Part model, mm, in its own coordinate system. A direction names the side the tool comes from. Coordinates: 2 decimals unless noted, no trailing zeros. Loops run counter-clockwise (first coordinate to the right, second up) from the corner with the lowest first, then second, coordinate; pieces in that order, holes last. Notation, with made-up numbers: (41.25, 20.25) - (55.25, 20.25) arc R35 ccw to (55.25, 58.25) - close; hole circle Ø4 at (-23.5, 49.5). An arc over 180 degrees is marked (long way). Use a Markdown table: item, result. Add a question column.
1. Band-saw the part on D-D, the plane x = 13. Give the cut face in (y, z).
2. Band-saw the part on C-C, the plane z = 9. Give the cut face in (x, y), plus the area to 3 significant figures.
3. Drop flat-ended pins along their axis: pin 1 (10 mm diameter, centred on y = -2, z = 5.5, fed in from -X); pin 2 (10 mm diameter, centred on x = -1, z = -10, fed in from -Y); pin 3 (1 mm diameter, centred on x = -7.5, z = -18.5, fed in from +Y); pin 4 (8 mm diameter, centred on y = -5.5, z = 2.5, fed in from -X). Give the stop position or say it passes through.
4. Band-saw the part on B-B, the plane y = -2. Give the cut face in (x, z), plus the area to 3 significant figures.
5. Band-saw the part on A-A, the plane x = -13. Give the cut face in (y, z), plus the area to 3 significant figures.
6. 3-axis set-ups, long thin cutter, end or side, ignore diameter. For faces 1 (the cylindrical face through (-15.95, -24.3, 18.51)), 2 (the flat face through (10, 1, 0)), 3 (the flat face through (-10, -7, 19)): which of +Z, -Z, +X, -X, +Y, -Y reach the whole face in a straight line?
7. Wall check: probe 1 along Y at (x, z) = (13, -18); probe 2 along Z at (x, y) = (1, -6); probe 3 along Y at (x, z) = (18, -17). Give the ranges that are in metal, low to high. Write a range as [from, to].
8. Pull direction Y, two halves, no side cores. Call faces 4 (the flat face through (0, -37, -18)), 5 (the flat face through (-5, 1.4, 4.4)), 6 (the cylindrical face through (12.479, -23.034, -18.486)), 7 (the flat face through (10, 3, 0)): pulls with the +Y half, pulls with the -Y half, needs draft (parallel to the pull), parting line crosses it, or undercut.
from build123d import *

# Parameters (mm, degrees)
HEAD_W_DEPTH        = 19.5
HEAD_T_W            = 35
HEAD_T_H            = 38
CUT_EXTRUDE_1_DEPTH = 66.186271561
SKETCH_3_R          = 4
CUT_EXTRUDE_2_DEPTH = 60.287435431


with BuildPart() as part:
    # ｽｹｯﾁ1 → Head-W (new, symmetric)
    with BuildSketch(Plane.XY):
        Polygon((-25, -37), (25, -37), (25, 3), (-5, 3), (-5, -7), (-15, -7), (-15, 3), (-25, 3), align=None)
    extrude(amount=HEAD_W_DEPTH, both=True)

    # Head-t → ｶｯﾄ - 押し出し1 (cut, through all)
    with BuildSketch(Plane(origin=(25, 0, 0), x_dir=(0, 0, -1), z_dir=(1, 0, 0))):
        with Locations((0, -18)):
            Rectangle(HEAD_T_W, HEAD_T_H)
    extrude(amount=-CUT_EXTRUDE_1_DEPTH, mode=Mode.SUBTRACT)

    # ｽｹｯﾁ3 → ｶｯﾄ - 押し出し2 (cut, through all)
    with BuildSketch(Plane.XY.offset(19.5)):
        with Locations((-13, -27)):
            Circle(SKETCH_3_R)
        with Locations((13, -27)):
            Circle(SKETCH_3_R)
    extrude(amount=-CUT_EXTRUDE_2_DEPTH, mode=Mode.SUBTRACT)


solid = part.part
Geometry check:
| question | item | result |
|---|---|---|
| 1 | outline | (-37, -19.5) - (-31, -19.5) - (-31, -17.5) - (-37, -17.5) - close; (-37, 17.5) - (-31, 17.5) - (-31, 19.5) - (-37, 19.5) - close; (-23, -19.5) - (3, -19.5) - (3, 19.5) - (-23, 19.5) - (-23, 17.5) - (1, 17.5) - (1, -17.5) - (-23, -17.5) - close |
| 2 | outline | (-25, 1) - (-15, 1) - (-15, 3) - (-25, 3) - close; (-5, 1) - (25, 1) - (25, 3) - (-5, 3) - close |
| 2 | area | 80.0 mm^2 |
| 3 | pin 1 | stops at x = -25 |
| 3 | pin 2 | stops at y = 1 |
| 3 | pin 3 | stops at y = -7 |
| 3 | pin 4 | passes through |
| 4 | outline | (-25, -19.5) - (-15, -19.5) - (-15, -17.5) - (-25, -17.5) - close; (-25, 17.5) - (-15, 17.5) - (-15, 19.5) - (-25, 19.5) - close; (-5, -19.5) - (25, -19.5) - (25, -17.5) - (-5, -17.5) - close; (-5, 17.5) - (25, 17.5) - (25, 19.5) - (-5, 19.5) - close |
| 4 | area | 160 mm^2 |
| 5 | outline | (-37, -19.5) - (-31, -19.5) - (-31, -17.5) - (-37, -17.5) - close; (-37, 17.5) - (-31, 17.5) - (-31, 19.5) - (-37, 19.5) - close; (-23, -19.5) - (-7, -19.5) - (-7, -17.5) - (-23, -17.5) - close; (-23, 17.5) - (-7, 17.5) - (-7, 19.5) - (-23, 19.5) - close |
| 5 | area | 88.0 mm^2 |
| 6 | face 1 | +Z, -Z |
| 6 | face 2 | +X, -X, -Y |
| 6 | face 3 | +Z, -Z, +Y |
| 7 | probe 1 | y = [-37, -31], [-23, 3] |
| 7 | probe 2 | z = [-19.5, -17.5], [17.5, 19.5] |
| 7 | probe 3 | y = [1, 3] |
| 8 | face 4 | pulls with the -Y half |
| 8 | face 5 | needs draft |
| 8 | face 6 | undercut |
| 8 | face 7 | pulls with the +Y half |
